Read the model definition and answer for the solid it produces. Units are mm, in the model's axes. Face numbers are marked on the shaded views. A direction names the side the tool comes from. Give positions to 0.01 mm unless a question says otherwise; leave off trailing zeros.
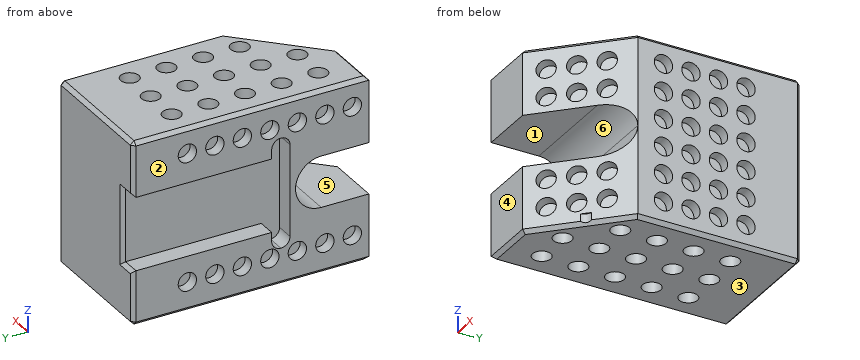
```python
from build123d import *

# Parameters (mm, degrees)
SKETCH1_W            = 35
SKETCH1_H            = 49.99
BOSS_EXTRUDE1_DEPTH  = 64.5
CUT_EXTRUDE1_REACH   = 85.46
CUT_EXTRUDE2_REACH   = 79.524
SKETCH3_W            = 14
SKETCH3_H            = 20
FILLET1_R            = 7
SKETCH4_W            = 5
SKETCH4_H            = 20
CUT_EXTRUDE3_DEPTH   = 43
SKETCH5_W            = 30
SKETCH5_H            = 5
CUT_EXTRUDE4_DEPTH   = 5
FILLET5_R            = 2.5
FILLET6_R            = 2.5
CHAMFER1_SIZE        = 1
SKETCH6_R            = 2.5
CUT_EXTRUDE5_DEPTH   = 3
LPATTERN1_COUNT      = 3
LPATTERN1_PITCH      = 10
LPATTERN1_COUNT_DIR2 = 5
LPATTERN1_PITCH_DIR2 = 10
SKETCH9_R            = 2.5
CUT_EXTRUDE20_DEPTH  = 3
LPATTERN2_COUNT      = 4
LPATTERN2_PITCH      = 7.5
LPATTERN2_COUNT_DIR2 = 6
LPATTERN2_PITCH_DIR2 = 7.5
SKETCH10_R           = 2.5
CUT_EXTRUDE21_DEPTH  = 3
LPATTERN3_COUNT      = 7
LPATTERN3_PITCH      = 7.5
LPATTERN3_COUNT_DIR2 = 2
LPATTERN3_PITCH_DIR2 = 35
SKETCH11_R           = 2.5
CUT_EXTRUDE23_DEPTH  = 3
LPATTERN5_COUNT      = 6
LPATTERN5_PITCH      = 7.5
LPATTERN5_COUNT_DIR2 = 3
LPATTERN5_PITCH_DIR2 = 7.5
CUT_EXTRUDE25_START  = -3
SKETCH18_R           = 2.5
CUT_EXTRUDE25_DEPTH  = 3
LPATTERN7_COUNT      = 3
LPATTERN7_PITCH      = 10
LPATTERN7_COUNT_DIR2 = 5
LPATTERN7_PITCH_DIR2 = 10


with BuildPart() as part:
    # Sketch1 → Boss-Extrude1 (new body)
    with BuildSketch(Plane(origin=(0, 0, 0), x_dir=(1, 0, 0), z_dir=(0, 1, 0))):
        Rectangle(SKETCH1_W, SKETCH1_H)
    extrude(amount=-BOSS_EXTRUDE1_DEPTH)

    # Sketch2 → Cut-Extrude1 (cut, up to next)
    with BuildSketch(Plane.XY.offset(24.995), mode=Mode.PRIVATE) as cut_extrude1_sk1:
        Polygon((-2.5, -64.5), (17.5, -44.5), (17.5, -64.5), align=None)
    cut_extrude1_tool1 = extrude(cut_extrude1_sk1.sketch, amount=-CUT_EXTRUDE1_REACH, mode=Mode.PRIVATE) & part.part
    add(cut_extrude1_tool1.solids().sort_by_distance((10.833333, -57.833333, 24.995))[0], mode=Mode.SUBTRACT)

    # Sketch3 → Cut-Extrude2 (cut, up to next)
    with BuildSketch(Plane.ZY.offset(17.5), mode=Mode.PRIVATE) as cut_extrude2_sk1:
        with Locations((0, -54.5)):
            Rectangle(SKETCH3_W, SKETCH3_H)
    cut_extrude2_tool1 = extrude(cut_extrude2_sk1.sketch, amount=-CUT_EXTRUDE2_REACH, mode=Mode.PRIVATE) & part.part
    add(cut_extrude2_tool1.solids().sort_by_distance((-17.5, -54.5, 0))[0], mode=Mode.SUBTRACT)

    # Fillet1
    fillet1_edges = [part.edges().sort_by_distance(p)[0] for p in [
        (0, -44.5, -7),
        (0, -44.5, 7),
    ]]
    fillet(fillet1_edges, radius=FILLET1_R - 0.0001)  # a hair under: the kernel refuses the full size

    # Sketch4 → Cut-Extrude3 (cut)
    with BuildSketch(Plane(origin=(0, 0, 0), x_dir=(1, 0, 0), z_dir=(0, 1, 0))):
        with Locations((-15, 0)):
            Rectangle(SKETCH4_W, SKETCH4_H)
    extrude(amount=-CUT_EXTRUDE3_DEPTH, mode=Mode.SUBTRACT)

    # Sketch5 → Cut-Extrude4 (cut)
    with BuildSketch(Plane.ZY.offset(17.5)):
        with Locations((0, -40.5)):
            Rectangle(SKETCH5_W, SKETCH5_H)
    extrude(amount=-CUT_EXTRUDE4_DEPTH, mode=Mode.SUBTRACT)

    # Fillet5
    fillet5_edges = [part.edges().sort_by_distance(p)[0] for p in [
        (-15, -38, -15),
        (-15, -43, -15),
    ]]
    fillet(fillet5_edges, radius=FILLET5_R - 0.0001)  # a hair under: the kernel refuses the full size

    # Fillet6
    fillet6_edges = [part.edges().sort_by_distance(p)[0] for p in [
        (-15, -43, 15),
        (-15, -38, 15),
    ]]
    fillet(fillet6_edges, radius=FILLET6_R - 0.0001)  # a hair under: the kernel refuses the full size

    # Chamfer1
    chamfer1_edges = [part.edges().sort_by_distance(p)[0] for p in [
        (-10, -64.5, -24.995),
        (17.5, -22.25, -24.995),
        (17.5, -22.25, 24.995),
        (-10, -64.5, 24.995),
        (7.5, -54.5, -24.995),
        (7.5, -54.5, 24.995),
        (0, 0, 24.995),
        (-17.5, 0, -17.4975),
        (-17.5, 0, 17.4975),
        (0, 0, -24.995),
        (17.5, 0, 0),
        (-15, 0, 10),
        (-12.5, 0, 0),
        (-15, 0, -10),
        (-17.5, -32.25, 24.995),
        (-17.5, -32.25, -24.995),
    ]]
    chamfer(chamfer1_edges, length=CHAMFER1_SIZE)

    # Sketch6 → Cut-Extrude5 (cut)
    with BuildSketch(Plane.XY.offset(24.995)):
        with Locations((-10, -15)):
            Circle(SKETCH6_R)
    cut_extrude5 = extrude(amount=-CUT_EXTRUDE5_DEPTH, mode=Mode.SUBTRACT)

    # LPattern1: Cut-Extrude5 3 × 5, 1 skipped
    with Locations(*[(i * LPATTERN1_PITCH, -j * LPATTERN1_PITCH_DIR2, 0) for i in range(LPATTERN1_COUNT) for j in range(LPATTERN1_COUNT_DIR2) if (i, j) not in ((0, 0), (2, 4))]):
        add(cut_extrude5, mode=Mode.SUBTRACT)

    # Sketch9 → Cut-Extrude20 (cut)
    with BuildSketch(Plane(origin=(17.5, 0, 0), x_dir=(0, 0, -1), z_dir=(1, 0, 0))):
        with Locations((-18.745, -15)):
            Circle(SKETCH9_R)
    cut_extrude20 = extrude(amount=-CUT_EXTRUDE20_DEPTH, mode=Mode.SUBTRACT)

    # LPattern2: Cut-Extrude20 4 × 6
    with Locations(*[(0, -i * LPATTERN2_PITCH, -j * LPATTERN2_PITCH_DIR2) for i in range(LPATTERN2_COUNT) for j in range(LPATTERN2_COUNT_DIR2) if (i, j) != (0, 0)]):
        add(cut_extrude20, mode=Mode.SUBTRACT)

    # Sketch10 → Cut-Extrude21 (cut)
    with BuildSketch(Plane.ZY.offset(17.5)):
        with Locations((-16.9975, -15)):
            Circle(SKETCH10_R)
    cut_extrude21 = extrude(amount=-CUT_EXTRUDE21_DEPTH, mode=Mode.SUBTRACT)

    # LPattern3: Cut-Extrude21 7 × 2
    with Locations(*[(0, -i * LPATTERN3_PITCH, j * LPATTERN3_PITCH_DIR2) for i in range(LPATTERN3_COUNT) for j in range(LPATTERN3_COUNT_DIR2) if (i, j) != (0, 0)]):
        add(cut_extrude21, mode=Mode.SUBTRACT)

    # Sketch11 → Cut-Extrude23 (cut)
    with BuildSketch(Plane(origin=(31, -31, 0), x_dir=(0, 0, -1), z_dir=(0.707106781186544, -0.7071067811865511, 0))):
        with Locations(Location((-18.745, -26.591883092, 0), (0, 0, 90))):
            Circle(SKETCH11_R)
    cut_extrude23 = extrude(amount=-CUT_EXTRUDE23_DEPTH, mode=Mode.SUBTRACT)

    # LPattern5: Cut-Extrude23 6 × 3, 6 skipped
    with Locations(*[Vector(0, 0, -1) * (i * LPATTERN5_PITCH) + Vector(-0.707106781186551, -0.707106781186544, 0) * (j * LPATTERN5_PITCH_DIR2) for i in range(LPATTERN5_COUNT) for j in range(LPATTERN5_COUNT_DIR2) if (i, j) not in ((0, 0), (2, 0), (2, 1), (2, 2), (3, 0), (3, 1), (3, 2))]):
        add(cut_extrude23, mode=Mode.SUBTRACT)

    # Sketch18 → Cut-Extrude25 (cut)
    with BuildSketch(Plane(origin=(0, 0, -24.995), x_dir=(-1, 0, 0), z_dir=(0, 0, -1)).offset(CUT_EXTRUDE25_START)):
        with Locations(Location((10, -15, 0), (0, 0, 180))):
            Circle(SKETCH18_R)
    cut_extrude25 = extrude(amount=CUT_EXTRUDE25_DEPTH, mode=Mode.SUBTRACT)

    # LPattern7: Cut-Extrude25 3 × 5
    with Locations(*[(i * LPATTERN7_PITCH, -j * LPATTERN7_PITCH_DIR2, 0) for i in range(LPATTERN7_COUNT) for j in range(LPATTERN7_COUNT_DIR2) if (i, j) != (0, 0)]):
        add(cut_extrude25, mode=Mode.SUBTRACT)


solid = part.part
```
Item 1: Each of these flat-tipped pins is pushed along its axis until it touches: pin 1 Ø4 at (y, z) = (-59.5, 17) entering from -X; pin 2 Ø8 at (y, z) = (-15, -3.755) entering from -X; pin 3 Ø4.5 at (y, z) = (-37.5, -17) entering from -X; pin 4 Ø4.5 at (y, z) = (-37.5, -18.755) entering from +X. Where does it stop, or does it pass through?
Result set:
pin 1: stops at x = -17.5
pin 2: stops at x = -12.5
pin 3: stops at x = -14.5
pin 4: stops at x = 14.5
Item 2: Section B-B (x = -1.5) is taken. Give the number of separate pieces and of enclosed holes in the cut face, and give its area (3 significant figures).
Result set:
separate pieces: 1
enclosed holes: 4
area: 2,790 mm2
Item 3: Find the intervals of material crossed by line 1 along Y through (x, z) = (-10, -23); line 2 along Z through (x, y) = (-15, -37) (3 decimals); line 3 along Y through (x, z) = (-14, 12), in increasing order.
Result set:
line 1: y = -64.5 to -57.5, -52.5 to -47.5, -42.5 to -37.5, -32.5 to -27.5, -22.5 to -17.5, -12.5 to 0
line 2: z = -24.995 to -19.447, -14.548 to -10, 10 to 15.553, 20.452 to 24.995
line 3: y = -64.5 to -43, -38 to 0
Item 4: Determine the mould class of the marked faces 3, 4, 5 and 6 for opening direction Z: pulls with the +Z half, pulls with the -Z half, needs draft (parallel to the pull), parting line crosses it, or undercut.
Result set:
face 3: pulls with the -Z half
face 4: needs draft
face 5: undercut
face 6: undercut
Item 5: Which of the six approach directions +Z, -Z, +X, -X, +Y, -Y give full straight-line access (tool end or side, diameter ignored) to the marked faces 1 and 2?
Result set:
face 1: +X, -X, -Y
face 2: +Z, -Z, -X, +Y, -Y
